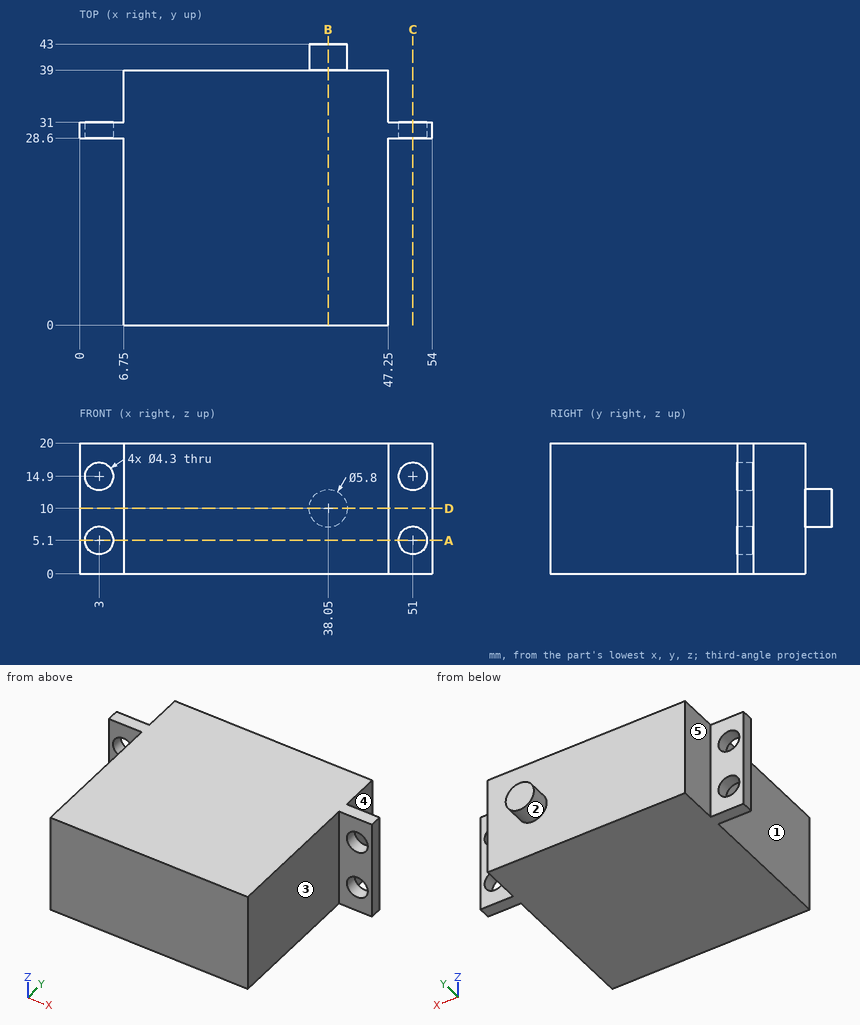
Job drawing, mm, ordinate dimensions from the low corner. One solid piece. A direction names the side the tool comes from. Give positions to 0.01 mm unless a question says otherwise; leave off trailing zeros. Loops run counter-clockwise (first coordinate to the right, second up) from the corner with the lowest first, then second, coordinate; pieces in that order, holes last. Notation, with made-up numbers: (-14.5, -25.75) - (-2.5, -25.75) arc R25 ccw to (-2.5, 0.25) - close; hole circle Ø9 at (57.5, 79.5). An arc over 180 degrees is marked (long way). Use one line per item in the form item = value.
(1) Drop flat-ended pins along their axis: P1, Ø3, axis at y = 10, z = 10, coming from the -X side; P2, Ø4, axis at y = 34.5, z = 11.5, coming from the +X side; P3, Ø10, axis at x = 29.5, z = 9.5, coming from the +Y side; P4, Ø7.5, axis at x = 49.5, z = 9, coming from the -Y side. Give the stop position or say it passes through.
Determined:
P1 = 6.75
P2 = 47.25
P3 = 39
P4 = 0
(2) Cut at A-A (z = 5.1). Give the cut face in (x, y), then the cut area to 3 significant figures.
Determined:
outline = (0, 28.6) - (0.85, 28.6) - (0.85, 31) - (0, 31) - close; (5.15, 28.6) - (6.75, 28.6) - (6.75, 0) - (47.25, 0) - (47.25, 28.6) - (48.85, 28.6) - (48.85, 31) - (47.25, 31) - (47.25, 39) - (6.75, 39) - (6.75, 31) - (5.15, 31) - close; (53.15, 28.6) - (54, 28.6) - (54, 31) - (53.15, 31) - close
area = 1,590 mm^2
(3) Cut at B-B (x = 38.05). Give the cut face in (y, z).
Determined:
outline = (0, 0) - (39, 0) - (39, 7.1) - (43, 7.1) - (43, 12.9) - (39, 12.9) - (39, 20) - (0, 20) - close
(4) 3-axis set-ups, long thin cutter, end or side, ignore diameter. For the marked faces 1, 2, 3, 4 and 5: which of +Z, -Z, +X, -X, +Y, -Y reach the whole face in a straight line?
Determined:
face_1 = +Z, -Z, -X, -Y
face_2 = +Y
face_3 = +Z, -Z, +X, -Y
face_4 = +Z, -Z, +X, +Y
face_5 = +Z, -Z, -X, +Y
(5) Cut at D-D (z = 10). Give the cut face in (x, y).
Determined:
outline = (0, 28.6) - (6.75, 28.6) - (6.75, 0) - (47.25, 0) - (47.25, 28.6) - (54, 28.6) - (54, 31) - (47.25, 31) - (47.25, 39) - (40.95, 39) - (40.95, 43) - (35.15, 43) - (35.15, 39) - (6.75, 39) - (6.75, 31) - (0, 31) - close
(6) Drill centre lines: L1, parallel to X at y = 30.2, z = 5.1; L2, parallel to Z at x = 51, y = 29.45; L3, parallel to Y at x = 36, z = 5. Where is each one in solid material? Low to high.
Determined:
L1 = 0 to 0.85, 5.15 to 48.85, 53.15 to 54
L2 = 0 to 2.95, 7.25 to 12.75, 17.05 to 20
L3 = 0 to 39
(7) Cut at C-C (x = 51). Give the cut face in (y, z).
Determined:
outline = (28.6, 0) - (31, 0) - (31, 2.95) - (28.6, 2.95) - close; (28.6, 7.25) - (31, 7.25) - (31, 12.75) - (28.6, 12.75) - close; (28.6, 17.05) - (31, 17.05) - (31, 20) - (28.6, 20) - close
